Design review of the part shown in the three views and the two pictorial views. Dimensions are in mm from the part's minimum x, y and z. Round coordinates to 2 decimals unless told otherwise and drop trailing zeros. Loops run counter-clockwise (first coordinate to the right, second up) from the corner with the lowest first, then second, coordinate; pieces in that order, holes last. Notation, with made-up numbers: M 40.25,44.5 L 63.25,44.5 A16 cw 63.25,66.5 Z; hole C -21,79.25 d5. An arc over 180 degrees is marked long. Return JSON: item names as keys, results as strings. Group by question number.
Q1. Consider section A-A (x = 47.5). State the section outline as (y, z) points, and give its area (3 significant figures).
Q2. To check wall thickness, follow line 1 along Y through (x, z) = (30.5, 2.2); line 2 along X through (y, z) = (44, 1.95); line 3 along Y through (x, z) = (16.5, 1.15). State the ranges of each line that lie inside material, in increasing order.
Q3. Clearance check with flat-ended pins moving along their axes: pin 1 Ø1.5 at (x, z) = (98, 1.5) entering from -Y; pin 2 Ø1 at (x, z) = (48.5, 0.5) entering from +Y; pin 3 Ø0.9 at (y, z) = (399, 1) entering from -X. State where each tip first meets the part, or that it passes through.
Q4. Consider section B-B (y = 136.5). State the section outline as (x, z) points.
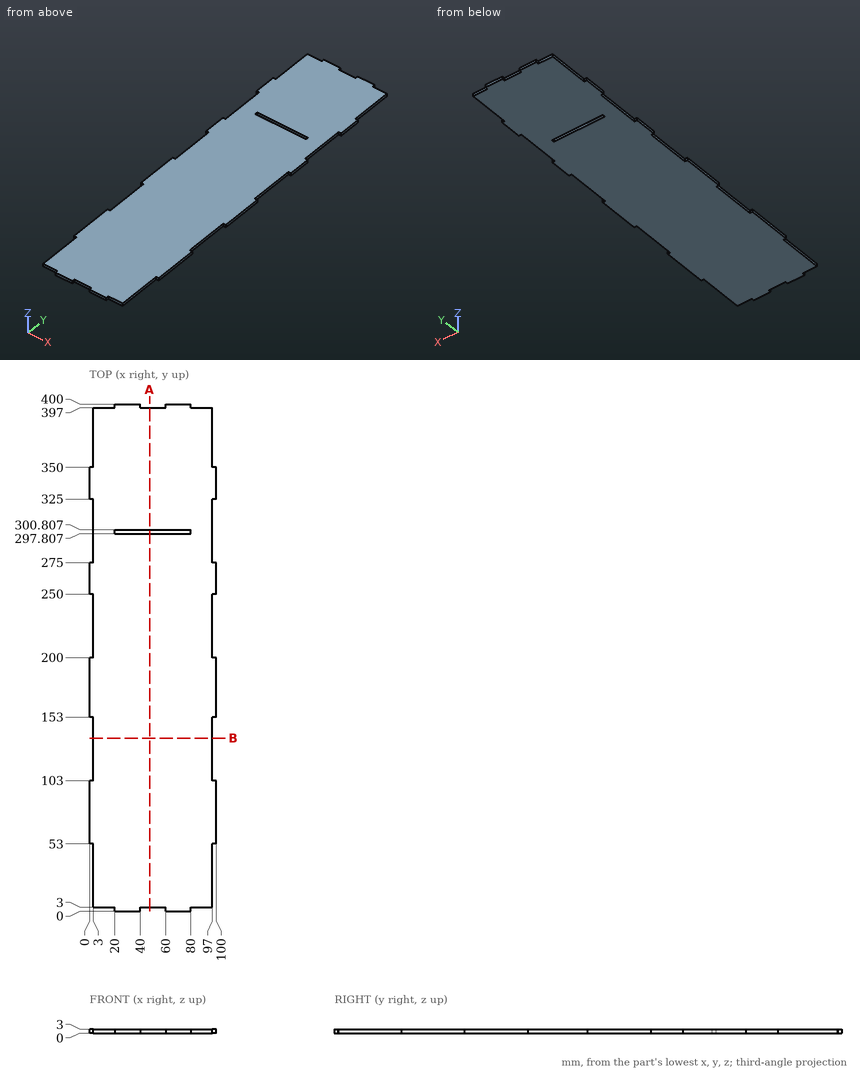
Values:
{
 "1": {"outline": "M 3,0 L 297.81,0 L 297.81,3 L 3,3 Z; M 300.81,0 L 397,0 L 397,3 L 300.81,3 Z", "area": "1,170 mm2"},
 "2": {"line 1": "y = 0 to 297.81, 300.81 to 400", "line 2": "x = 3 to 97", "line 3": "y = 3 to 397"},
 "3": {"pin 1": "stops at y = 53", "pin 2": "stops at y = 397", "pin 3": "stops at x = 20"},
 "4": {"outline": "M 3,0 L 97,0 L 97,3 L 3,3 Z"}
}
